CAD build for the part. Positions are in the model's coordinates, mm. A direction names the side the tool comes from. Coordinates: 2 decimals unless noted, no trailing zeros. Order: outer loops, then holes, each group sorted by start corner. A loop starts at its lowest first (then second) coordinate and runs counter-clockwise, first axis right, second up. Notation, with made-up numbers: (9.5, -32.75) -> (23.5, -32.75) arc R20 cw to (23.5, -9.75) -> close; hole circle Ø5 at (75, 43). An arc over 180 degrees is marked (long way). Use one line per item in the form item = value. Start each with the question number.
Autodesk Inventor part; units mm, degrees
ref_plane "YZ Plane" through (0, 0, 0) normal (1, 0, 0) x (0, 1, 0)
ref_plane "XZ Plane" through (0, 0, 0) normal (0, 1, 0) x (-1, 0, 0)
ref_plane "XY Plane" through (0, 0, 0) normal (0, 0, 1) x (1, 0, 0)
sketch "Sketch2" plane through (0, 0, 0) normal (0, 0, 1) x (1, 0, 0)
  circle A0 centre (0, 0) radius 6
  dimension "d3" = 12
extrude "Extrusion2" add sketch "Sketch2" along normal blind 11.5
sketch "Sketch3" plane through (0, 0, 11.5) normal (0, 0, 1) x (1, 0, 0)
  line L0 (-3.476, 6) -> (3.4581, 6.0103)
  line L1 (3.4581, 6.0103) -> (6.9342, 0.0103)
  line L2 (6.9342, 0.0103) -> (3.476, -6)
  line L3 (3.476, -6) -> (-3.4581, -6.0103)
  line L4 (-3.4581, -6.0103) -> (-6.9342, -0.0103)
  line L5 (-6.9342, -0.0103) -> (-3.476, 6)
  point P0 (0, 0)
  point P1 (0, 0)
sketch "Sketch4" plane through (0, 0, 0) normal (0, 0, -1) x (-1, 0, 0)
  circle A0 centre (0, 0) radius 3
  dimension "d6" = 6
extrude "Extrusion3" add sketch "Sketch3" along normal blind 6
extrude "Extrusion4" cut sketch "Sketch4" against normal up to surface (11.5 mm away)
sketch "Sketch5" plane through (-3.476, 6, 17.5) normal (-0.0014906, 0.9999989, 0) x (0.9999989, 0.0014906, 0)
  line L0 (0, 0) -> (-3.4671, 0)
  line L1 (6.9342, 6) -> (6.9342, 0)
  line L2 (0, 0) -> (6.9342, 0)
  line L3 (6.9342, 0) -> (6.9342, 6)
  line L4 (6.9342, 6) -> (0, 6)
  line L5 (0, 6) -> (0, 0)
  line L6 (3.4671, 0) -> (3.4671, 17.5) construction
  line L7 (6.9342, 6) -> (0, 6) construction
  line L8 (6.9342, 6) -> (0, 6) construction
  circle A0 centre (3.4671, 11.75) radius 1.5
  dimension "d11" = 3
extrude "Extrusion5" cut sketch "Sketch5" against normal through all contours A0
sketch "Sketch6" plane through (0, 0, 17.5) normal (0, 0, 1) x (1, 0, 0)
  circle A0 centre (0, 0) radius 1.5
  dimension "d14" = 3
extrude "Extrusion6" cut sketch "Sketch6" against normal blind 10
properties part number "Wheel Test" material "Brass"
1) 3-axis set-ups, long thin cutter, end or side, ignore diameter. For faces 1 (the face through (-5.172, -3.052, 14.458)), 2 (the face through (6.1, 0.9, 11.5)): which of +Z, -Z, +X, -X, +Y, -Y reach the whole face in a straight line?
2) Cut at D-D on y = 2. Give the cut face in (x, z).
3) Cut at A-A on z = 15.25. Give the cut face in (x, y), then the cut area to 3 significant figures.
4) Drop flat-ended pins along their axis: P1, Ø6, axis at x = 3, y = -2.5, coming from the -Z side; P2, Ø1, axis at y = -0.5, z = 6.5, coming from the -X side; P3, Ø1.5, axis at y = -2.5, z = 10.5, coming from the -X side; P4, Ø1, axis at y = 4.5, z = 6.5, coming from the +X side. Give the stop position or say it passes through.
5) Two-plate mould, pull along Z, no slides. Class faces 3 (the face through (-2.77, -1.15, 5.67)), 4 (the face through (-0.319, -4.276, 7.214)), 5 (the face through (1.4, 1.4, 17.5)), 6 (the face through (-1.2, 4.32, 6.66)): released by +Z, released by -Z, zero draft, split by the parting line, or undercut.
6) Cut at C-C on x = -4. Give the cut face in (y, z).
7) Cut at B-B on y = 0.5. Give the cut face in (x, z).
8) Probe L1, parallel to Y at x = 0, z = 15.5; L2, parallel to Y at x = -0.75, z = 13.25; L3, parallel to X at y = -1.25, z = 2.75. List the from-to ranges inside material, lowest first.
Values follow:
q1.face_1 = +Z, -Z, -X, -Y
q1.face_2 = -Z
q2.outline = (-5.78, 11.5) -> (-5.66, 11.5) -> (-5.66, 0) -> (-2.24, 0) -> (-2.24, 11.5) -> (2.24, 11.5) -> (2.24, 0) -> (5.66, 0) -> (5.66, 11.5) -> (5.78, 11.5) -> (5.78, 17.5) -> (-5.78, 17.5) -> close
q3.outline = (-6.93, -0.01) -> (-3.46, -6.01) -> (3.48, -6) -> (6.93, 0.01) -> (3.46, 6.01) -> (-3.48, 6) -> close; hole circle Ø3 at (0, 0)
q3.area = 118 mm^2
q4.P1 = 0
q4.P2 = -6
q4.P3 = -5.74
q4.P4 = 4.47
q5.face_3 = zero draft
q5.face_4 = undercut
q5.face_5 = released by +Z
q5.face_6 = undercut
q6.outline = (-5.07, 11.5) -> (-4.47, 11.5) -> (-4.47, 0) -> (4.47, 0) -> (4.47, 11.5) -> (5.09, 11.5) -> (5.09, 17.5) -> (-5.07, 17.5) -> close
q7.outline = (-6.64, 11.5) -> (-5.98, 11.5) -> (-5.98, 0) -> (-2.96, 0) -> (-2.96, 11.5) -> (-1.41, 11.5) -> (-1.41, 17.5) -> (-6.64, 17.5) -> close; (1.41, 11.5) -> (2.96, 11.5) -> (2.96, 0) -> (5.98, 0) -> (5.98, 11.5) -> (6.65, 11.5) -> (6.65, 17.5) -> (1.41, 17.5) -> close
q8.L1 = -6.01 to -1.5, 1.5 to 6.01
q8.L2 = -6.01 to -1.3, 1.3 to 6
q8.L3 = -5.87 to -2.73, 2.73 to 5.87
